from build123d import *

# Parameters (mm, degrees)
F0_W     = 100
F0_H     = 100
F0_W_2   = 94
F0_H_2   = 94
F1_DEPTH = 950
F3_DEPTH = 100
F5_DEPTH = 100


with BuildPart() as f1:
    # F0 (on Top) → F1 (new body)
    with BuildSketch(Plane.XY):
        with Locations((3.593751, -13.807164)):
            Rectangle(F0_W, F0_H)
        with Locations((3.593751, -13.807164)):
            Rectangle(F0_W_2, F0_H_2, mode=Mode.SUBTRACT)
    extrude(amount=F1_DEPTH)

    # F2 (on face) → F3 (cut)
    with BuildSketch(Plane.XZ.offset(63.807164)):
        Polygon((-46.406249, 850), (53.593751, 950), (-46.406249, 950), align=None)
    extrude(amount=-F3_DEPTH, mode=Mode.SUBTRACT)

    # F4 (on face) → F5 (cut)
    with BuildSketch(Plane.XZ.offset(63.807164)):
        Polygon((-46.406249, 0), (53.593751, 0), (-46.406249, 100), align=None)
    extrude(amount=-F5_DEPTH, mode=Mode.SUBTRACT)


solid = f1.part
Can you work these out from the model? Positions are in its coordinate system, mm. A direction names the side the tool comes from. Round coordinates to 2 decimals unless told otherwise and drop trailing zeros. Write each loop counter-clockwise with the first axis right and the second up, starting at its lowest first coordinate (ties: lowest second). Pieces come first, ordered by that corner, then holes. Notation, with made-up numbers: M 22.25,12 L 67.25,12 A12 cw 67.25,19 Z; hole C 17,51.5 d3. An arc over 180 degrees is marked long. Use a Markdown table: item, result.
Item 1: I want a section at B-B (x = -14.5). List the corners of the cut face in (y, z) for me, and give its area (3 significant figures).
Found:
| item | result |
|---|---|
| outline | M -63.81,68.09 L -60.81,68.09 L -60.81,881.91 L -63.81,881.91 Z; M 33.19,68.09 L 36.19,68.09 L 36.19,881.91 L 33.19,881.91 Z |
| area | 4,880 mm2 |
Item 2: We'd pull the mould along X, two halves only. Please class faces 3 (the face through (-46.406, -15, 470)), 4 (the face through (3, 33.193, 468)), 5 (the face through (3, 36.193, 468)): released by +X, released by -X, zero draft, split by the parting line, or undercut.
Found:
| item | result |
|---|---|
| face 3 | released by -X |
| face 4 | undercut |
| face 5 | zero draft |
Item 3: I want a section at C-C (z = 748). List the corners of the cut face in (x, y) for me, and give its area (3 significant figures).
Found:
| item | result |
|---|---|
| outline | M -46.41,-63.81 L 53.59,-63.81 L 53.59,36.19 L -46.41,36.19 Z; hole M -43.41,-60.81 L 50.59,-60.81 L 50.59,33.19 L -43.41,33.19 Z |
| area | 1,160 mm2 |
Item 4: I want a section at D-D (z = 865). List the corners of the cut face in (x, y) for me.
Found:
| item | result |
|---|---|
| outline | M -31.41,-63.81 L 53.59,-63.81 L 53.59,36.19 L -31.41,36.19 L -31.41,33.19 L 50.59,33.19 L 50.59,-60.81 L -31.41,-60.81 Z |
Item 5: I want a section at A-A (y = -39.5). List the corners of the cut face in (x, z) for me, and give its area (3 significant figures).
Found:
| item | result |
|---|---|
| outline | M -46.41,100 L -43.41,97 L -43.41,853 L -46.41,850 Z; M 50.59,3 L 53.59,0 L 53.59,950 L 50.59,947 Z |
| area | 5,100 mm2 |
Item 6: If I drill on line 1 along Y through (x, z) = (16, 265); line 2 along X through (y, z) = (19.5, 719.5); line 3 along X through (y, z) = (32.5, 886), over which ranges is the centre line in solid material (lowest first)? Write a range as [from, to].
Found:
| item | result |
|---|---|
| line 1 | y = [-63.81, -60.81], [33.19, 36.19] |
| line 2 | x = [-46.41, -43.41], [50.59, 53.59] |
| line 3 | x = [50.59, 53.59] |
Item 7: Which directions (+Z, -Z, +X, -X, +Y, -Y) give clear straight access to the entire face, cutting with the end or side of a thin tool? Please do faces 1 (the face through (50.594, -14, 468)), 2 (the face through (7.531, 34.108, 46.063)).
Found:
| item | result |
|---|---|
| face 1 | +Z, -Z |
| face 2 | -Z, -X, +Y, -Y |
